Part model, mm, in its own coordinate system. Face numbers are marked on the shaded views. Round coordinates to 2 decimals unless told otherwise and drop trailing zeros. Order: outer loops, then holes, each group sorted by start corner. A loop starts at its lowest first (then second) coordinate and runs counter-clockwise, first axis right, second up. Notation, with made-up numbers: (16.25, 26) - (69.25, 26) arc R23 cw to (69.25, 51) - close; hole circle Ø2 at (7, 61). An arc over 180 degrees is marked (long way). Answer as a JSON object with one key per item and string values.
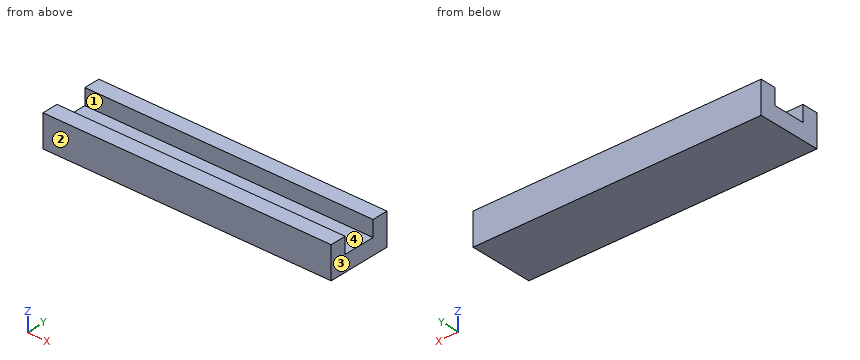
```python
from build123d import *

# Parameters (mm, degrees)
BOSS_EXTRUDE1_DEPTH = 10
CUT_EXTRUDE2_DEPTH  = 22
BOSS_EXTRUDE2_DEPTH = 5


with BuildPart() as part:
    # Sketch1 → Boss-Extrude1 (new body)
    with BuildSketch(Plane.XY):
        Polygon((45, 0), (45, 10), (-45, 10), (-45, 0), (-45, -10), (45, -10), align=None)
    extrude(amount=BOSS_EXTRUDE1_DEPTH)

    # Sketch2 → Cut-Extrude2 (cut)
    with BuildSketch(Plane.XY):
        Polygon((0, 5), (45, 5), (45, -5), (0, -5), (-45, -5), (-45, 5), align=None)
    extrude(amount=CUT_EXTRUDE2_DEPTH, mode=Mode.SUBTRACT)


with BuildPart() as cut_extrude2_piece_1:
    # of the separate pieces the step leaves, piece 1, a body of its own (cut_extrude2_pieces)
    add(part.part.solids().sort_by_distance((45, -5, 0))[0])



with BuildPart() as cut_extrude2_piece_2:
    # of the separate pieces the step leaves, piece 2, a body of its own (cut_extrude2_pieces)
    add(part.part.solids().sort_by_distance((45, 10, 0))[0])


with BuildPart() as cut_extrude2_piece_1_1:
    add(cut_extrude2_piece_1.part)

    add(cut_extrude2_piece_2.part)  # Boss-Extrude2 merges Cut-Extrude2 piece 2
    # Sketch2<3> → Boss-Extrude2 (add)
    with BuildSketch(Plane.XY):
        Polygon((0, 5), (45, 5), (45, -5), (0, -5), (-45, -5), (-45, 5), align=None)
    extrude(amount=BOSS_EXTRUDE2_DEPTH)


solid = cut_extrude2_piece_1_1.part
```
Item 1: Drop a flat-ended pin along its axis: P1, Ø8, axis at x = 6, y = -0.5, coming from the +Z side. Give the stop position or say it passes through.
Taken from the geometry:
{"P1": "z = 5"}
Item 2: Probe L1, parallel to Y at x = 16, z = 7; L2, parallel to Z at x = -37, y = 1.75. List the from-to ranges inside material, lowest first. Write a range as from..to.
Taken from the geometry:
{"L1": "-10..-5, 5..10", "L2": "0..5"}
Item 3: Cut at A-A (z = 8.75). Write the cut outline in (x, y), plus the area to 3 significant figures.
Taken from the geometry:
{"outline": "(-45, -10) - (45, -10) - (45, -5) - (-45, -5) - close; (-45, 5) - (45, 5) - (45, 10) - (-45, 10) - close", "area": "900 mm2"}
Item 4: Two-plate mould, pull along Y, no slides. Class the marked faces 1, 2, 3 and 4: pulls with the +Y half, pulls with the -Y half, needs draft (parallel to the pull), parting line crosses it, or undercut.
Taken from the geometry:
{"face 1": "undercut", "face 2": "pulls with the -Y half", "face 3": "needs draft", "face 4": "undercut"}
Item 5: Cut at C-C (y = 2). Write the cut outline in (x, z).
Taken from the geometry:
{"outline": "(-45, 0) - (45, 0) - (45, 5) - (-45, 5) - close"}
Item 6: Cut at B-B (x = 12.5). Write the cut outline in (y, z), plus the area to 3 significant figures.
Taken from the geometry:
{"outline": "(-10, 0) - (10, 0) - (10, 10) - (5, 10) - (5, 5) - (-5, 5) - (-5, 10) - (-10, 10) - close", "area": "150 mm2"}
